Design review of the part built by this model. Coordinates are the model's own, in mm. A direction names the side the tool comes from. Give positions to 0.01 mm unless a question says otherwise; leave off trailing zeros. Write each loop counter-clockwise with the first axis right and the second up, starting at its lowest first coordinate (ties: lowest second). Pieces come first, ordered by that corner, then holes. Notation, with made-up numbers: (60, 31.5) -> (115, 31.5) arc R29 cw to (115, 67.5) -> close; hole circle Ø4 at (-36.5, 26). An arc over 180 degrees is marked (long way). Use CSV: the item, a comma, the result in double quotes.
```python
from build123d import *

# Parameters (mm, degrees)
SKETCH1_W           = 19.56
SKETCH1_H           = 40.64
BOSS_EXTRUDE1_DEPTH = 37.96
SKETCH2_W           = 53.34
SKETCH2_H           = 2.5
BOSS_EXTRUDE2_DEPTH = 19.56
SKETCH3_R           = 2.195
CUT_EXTRUDE1_DEPTH  = 30.44
SKETCH4_W           = 2.5
SKETCH4_H           = 0.665692654
CUT_EXTRUDE2_DEPTH  = 30.44
SKETCH5_R           = 6
BOSS_EXTRUDE3_DEPTH = 3.15
SKETCH6_R           = 12
BOSS_EXTRUDE4_DEPTH = 3.2
SKETCH7_R           = 1.25
CUT_EXTRUDE3_DEPTH  = 3.2
SKETCH8_R           = 3.685
BOSS_EXTRUDE5_DEPTH = 4.06


with BuildPart() as part:
    # Sketch1 → Boss-Extrude1 (new body)
    with BuildSketch(Plane(origin=(0, 0, 0), x_dir=(1, 0, 0), z_dir=(0, 1, 0))):
        Rectangle(SKETCH1_W, SKETCH1_H)
    extrude(amount=BOSS_EXTRUDE1_DEPTH)

    # Sketch2 → Boss-Extrude2 (add)
    with BuildSketch(Plane(origin=(9.78, 0, 0), x_dir=(0, 0, -1), z_dir=(1, 0, 0))):
        with Locations((0, 28.19)):
            Rectangle(SKETCH2_W, SKETCH2_H)
    extrude(amount=-BOSS_EXTRUDE2_DEPTH)

    # Sketch3 → Cut-Extrude1 (cut, through all)
    with BuildSketch(Plane(origin=(0, 29.44, 0), x_dir=(1, 0, 0), z_dir=(0, 1, 0))):
        with Locations((-5.1, 24.2)):
            Circle(SKETCH3_R)
        with Locations((5.1, 24.2)):
            Circle(SKETCH3_R)
        with Locations((5.1, -24.2)):
            Circle(SKETCH3_R)
        with Locations((-5.1, -24.2)):
            Circle(SKETCH3_R)
    extrude(amount=-CUT_EXTRUDE1_DEPTH, mode=Mode.SUBTRACT)

    # Sketch4 → Cut-Extrude2 (cut, through all)
    with BuildSketch(Plane(origin=(0, 29.44, 0), x_dir=(1, 0, 0), z_dir=(0, 1, 0))):
        with Locations((5.1, 26.337153673)):
            Rectangle(SKETCH4_W, SKETCH4_H)
        with Locations((-5.1, 26.337153673)):
            Rectangle(SKETCH4_W, SKETCH4_H)
        with Locations((5.1, -26.337153673)):
            Rectangle(SKETCH4_W, SKETCH4_H)
        with Locations((-5.1, -26.337153673)):
            Rectangle(SKETCH4_W, SKETCH4_H)
    extrude(amount=-CUT_EXTRUDE2_DEPTH, mode=Mode.SUBTRACT)

    # Sketch5 → Boss-Extrude3 (add)
    with BuildSketch(Plane(origin=(0, 37.96, 0), x_dir=(1, 0, 0), z_dir=(0, 1, 0))):
        with Locations((0, 10.39)):
            Circle(SKETCH5_R)
    extrude(amount=BOSS_EXTRUDE3_DEPTH)

    # Sketch6 → Boss-Extrude4 (add)
    with BuildSketch(Plane(origin=(0, 41.11, 0), x_dir=(1, 0, 0), z_dir=(0, 1, 0))):
        with Locations((0, 10.39)):
            Circle(SKETCH6_R)
    extrude(amount=BOSS_EXTRUDE4_DEPTH)

    # Sketch7 → Cut-Extrude3 (cut)
    with BuildSketch(Plane(origin=(0, 44.31, 0), x_dir=(1, 0, 0), z_dir=(0, 1, 0))):
        with Locations((0, 18.72)):
            Circle(SKETCH7_R)
        with Locations((5.890199487, 16.280199487)):
            Circle(SKETCH7_R)
        with Locations((8.33, 10.39)):
            Circle(SKETCH7_R)
        with Locations((5.890199487, 4.499800513)):
            Circle(SKETCH7_R)
        with Locations((0, 2.06)):
            Circle(SKETCH7_R)
        with Locations((-5.890199487, 4.499800513)):
            Circle(SKETCH7_R)
        with Locations((-8.33, 10.39)):
            Circle(SKETCH7_R)
        with Locations((-5.890199487, 16.280199487)):
            Circle(SKETCH7_R)
    extrude(amount=-CUT_EXTRUDE3_DEPTH, mode=Mode.SUBTRACT)

    # Sketch8 → Boss-Extrude5 (add)
    with BuildSketch(Plane.XZ):
        with Locations((0, -10.39)):
            Circle(SKETCH8_R)
    extrude(amount=BOSS_EXTRUDE5_DEPTH)


solid = part.part
```
(1) Tool access review of faces 5 (the face through (0.672, 42.732, -19.774)), 6 (the face through (0, 29.44, 24)), 7 (the face through (-6, 41.11, -8)), 8 (the face through (1.98, -2, -7.28)): name each direction out of +Z, -Z, +X, -X, +Y, -Y from which nothing blocks a thin tool from reaching the whole face with its end or side.
Established:
face 5,"+Y"
face 6,"+Z, +X, -X, +Y"
face 7,"none"
face 8,"-Y"
(2) Take a section at A-A (z = -24.2). Write out the cut boundary in (x, y) (3 decimals), then the cut area to 4 significant figures.
Established:
outline,"(-9.78, 26.94) -> (-7.295, 26.94) -> (-7.295, 29.44) -> (-9.78, 29.44) -> close; (-2.905, 26.94) -> (2.905, 26.94) -> (2.905, 29.44) -> (-2.905, 29.44) -> close; (7.295, 26.94) -> (9.78, 26.94) -> (9.78, 29.44) -> (7.295, 29.44) -> close"
area,"26.95 mm2"
(3) For line 1 along Z through (x, y) = (0, 42); line 2 along X through (y, z) = (42.75, -10.39); line 3 along Y through (x, z) = (-7, -6.5), list the stretches that pass through material, from the lowest coordinate up. Write a range as [from, to].
Established:
line 1,"z = [-22.39, -19.97], [-17.47, -3.31], [-0.81, 1.61]"
line 2,"x = [-12, -9.58], [-7.08, 7.08], [9.58, 12]"
line 3,"y = [0, 37.96], [41.11, 44.31]"
(4) Take a section at C-C (z = -10.39). Write out the cut boundary in (x, y) (3 decimals).
Established:
outline,"(-12, 41.11) -> (-9.58, 41.11) -> (-9.58, 44.31) -> (-12, 44.31) -> close; (-9.78, 0) -> (-3.685, 0) -> (-3.685, -4.06) -> (3.685, -4.06) -> (3.685, 0) -> (9.78, 0) -> (9.78, 37.96) -> (6, 37.96) -> (6, 41.11) -> (7.08, 41.11) -> (7.08, 44.31) -> (-7.08, 44.31) -> (-7.08, 41.11) -> (-6, 41.11) -> (-6, 37.96) -> (-9.78, 37.96) -> close; (9.58, 41.11) -> (12, 41.11) -> (12, 44.31) -> (9.58, 44.31) -> close"
(5) Clearance check with flat-ended pins moving along their axes: pin 1 (3.5 mm diameter, centred on x = 5.1, z = 24.2, fed in from +Y); pin 2 (1 mm diameter, centred on y = 9.5, z = -7.5, fed in from -X); pin 3 (3 mm diameter, centred on x = -8.33, z = -10.39, fed in from -Y); pin 4 (7 mm diameter, centred on x = -3.5, z = 24.5, fed in from +Y). State where each tip first meets the part, or that it passes through.
Established:
pin 1,"passes through"
pin 2,"stops at x = -9.78"
pin 3,"stops at y = 0"
pin 4,"stops at y = 29.44"
(6) Take a section at D-D (y = 39). Write out the cut boundary in (x, z).
Established:
outline,"circle Ø12 at (0, -10.39)"
(7) Take a section at B-B (x = 0). State how many separate pieces and enclosed holes the cut face has, then the cut area to 3 significant figures.
Established:
separate pieces,"3"
enclosed holes,"0"
area,"1,700 mm2"
(8) Mouldability with a two-part tool opening along Y and no side actions: class faces 1 (the face through (-4.42, 39.51, -14.45)), 2 (the face through (0, 28, 26.67)), 3 (the face through (0, 0, 0)), 4 (the face through (0, 34, -20.32)) as +Y half, -Y half, draft (parallel to the pull), parting line (faces both ways), or undercut.
Established:
face 1,"undercut"
face 2,"draft"
face 3,"-Y half"
face 4,"undercut"
